from build123d import *

# Parameters (mm, degrees)
F0_R     = 7.2809687116
F0_R_2   = 7.0556428797
F1_DEPTH = 20
F2_R     = 9.99999


# Not quite as in the source:
# - a fillet or chamfer is up to 0.001 mm smaller than in the source, because OpenCascade refuses the exact size


with BuildPart() as f1:
    # F0 (on Top) → F1 (new body)
    with BuildSketch(Plane.XY):
        Polygon((-20, 20), (-20, 0), (-20, -20), (-10, -20), (-10, -60), (10, -60), (10, -20), (20.4342082143, -20), (20.4342082143, 20), (10, 20), (10, 60), (-10, 60), (-10, 20), align=None)
        with Locations((0, -50.0781983137)):
            Circle(F0_R, mode=Mode.SUBTRACT)
        with Locations((0, 49.5025888085)):
            Circle(F0_R_2, mode=Mode.SUBTRACT)
    extrude(amount=F1_DEPTH)

    # F2 (radius 10 in the source; OpenCascade refuses exactly that, so slightly less here)
    f2_edges = [f1.edges().sort_by_distance(p)[0] for p in [
        (10, 60, 10),
        (-10, 60, 10),
        (10, -60, 10),
        (-10, -60, 10),
    ]]
    fillet(f2_edges, radius=F2_R)


solid = f1.part
The listing builds one solid part. Answer for the finished solid, in the listing's coordinates (mm). A direction names the side the tool comes from. Give positions to 0.01 mm unless a question says otherwise; leave off trailing zeros. Loops run counter-clockwise (first coordinate to the right, second up) from the corner with the lowest first, then second, coordinate; pieces in that order, holes last.
Item 1: Find the intervals of material crossed by line 1 along Y through (x, z) = (0, 12.25); line 2 along Y through (x, z) = (0.5, 6.25); line 3 along X through (y, z) = (49.5, 14.5), in increasing order.
Derived:
line 1: y = -60 to -57.36, -42.8 to 42.45, 56.56 to 60
line 2: y = -59.99 to -57.34, -42.81 to 42.46, 56.54 to 59.99
line 3: x = -10 to -7.06, 7.06 to 10
Item 2: Each of these flat-tipped pins is pushed along its axis until it touches: pin 1 Ø5 at (x, z) = (13.5, 6) entering from +Y; pin 2 Ø10 at (x, y) = (2, 37.5) entering from -Z; pin 3 Ø5 at (x, z) = (-15, 14.5) entering from -Y; pin 4 Ø6 at (y, z) = (-39.5, 11) entering from -X. Where does it stop, or does it pass through?
Derived:
pin 1: stops at y = 20
pin 2: stops at z = 0
pin 3: stops at y = -20
pin 4: stops at x = -10
Item 3: A cutting plane is placed at C-C (x = -12.5). Give the vertices of the cut face in (y, z).
Derived:
outline: (-20, 0) - (20, 0) - (20, 20) - (-20, 20) - close
Item 4: A cutting plane is placed at A-A (y = 47). Give the vertices of the cut face in (x, z), then the cut area to 3 significant figures.
Derived:
outline: (-10, 0) - (-6.6, 0) - (-6.6, 20) - (-10, 20) - close; (6.6, 0) - (10, 0) - (10, 20) - (6.6, 20) - close
area: 136 mm2
Item 5: A tool of negligible diameter and unlimited length cuts with its end or side. For faces 1 (the flat face through (-10, -35, 10)), 2 (the flat face through (10, -35, 10)), 3 (the flat face through (-10, 35, 10)), 4 (the flat face through (15, 20, 10)), from which of +Z, -Z, +X, -X, +Y, -Y can it reach the whole face along a straight path? Write none if from no direction.
Derived:
face 1: +Z, -Z, -X, -Y
face 2: +Z, -Z, +X, -Y
face 3: +Z, -Z, -X, +Y
face 4: +Z, -Z, +X, +Y
Item 6: A cutting plane is placed at B-B (z = 2.75). Give the number of separate pieces and of enclosed holes in the cut face, then the cut area to 3 significant figures.
Derived:
separate pieces: 1
enclosed holes: 2
area: 2,810 mm2
Item 7: A cutting plane is placed at D-D (y = -48). Give the vertices of the cut face in (x, z), then the cut area to 3 significant figures.
Derived:
outline: (-10, 0) - (-6.98, 0) - (-6.98, 20) - (-10, 20) - close; (6.98, 0) - (10, 0) - (10, 20) - (6.98, 20) - close
area: 121 mm2
Item 8: Determine the mould class of faces 5 (the cylindrical face through (3.793, 55.452, 9.86)), 6 (the flat face through (15, -20, 10)), 7 (the flat face through (20.434, 0, 10)) for opening direction X: +X half, -X half, draft (parallel to the pull), parting line (faces both ways), or undercut.
Derived:
face 5: undercut
face 6: draft
face 7: +X half
